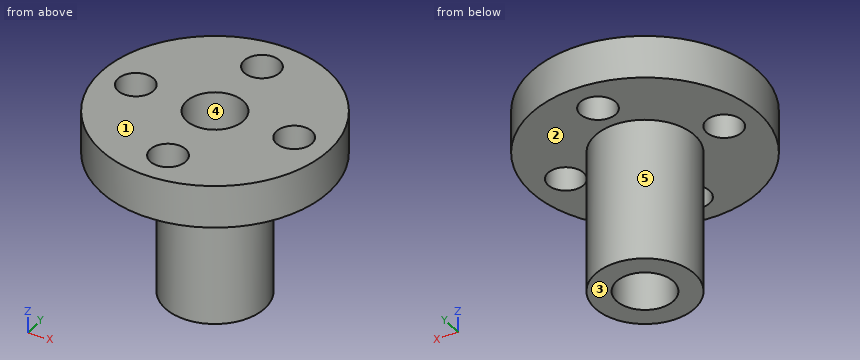
from build123d import *

# Parameters (mm, degrees)
SKETCH1_R           = 8
SKETCH1_R_2         = 1.25
BOSS_EXTRUDE1_DEPTH = 3
SKETCH2_R           = 3.5
BOSS_EXTRUDE2_DEPTH = 10
SKETCH3_R           = 2
CUT_EXTRUDE1_DEPTH  = 18.23368794


with BuildPart() as part:
    # Sketch1 → Boss-Extrude1 (new body)
    with BuildSketch(Plane.XY):
        Circle(SKETCH1_R)
        with Locations((0, 5.5)):
            Circle(SKETCH1_R_2, mode=Mode.SUBTRACT)
        with Locations((5.5, 0)):
            Circle(SKETCH1_R_2, mode=Mode.SUBTRACT)
        with Locations((0, -5.5)):
            Circle(SKETCH1_R_2, mode=Mode.SUBTRACT)
        with Locations((-5.5, 0)):
            Circle(SKETCH1_R_2, mode=Mode.SUBTRACT)
    extrude(amount=BOSS_EXTRUDE1_DEPTH)

    # Sketch2 → Boss-Extrude2 (add)
    with BuildSketch(Plane.XY):
        Circle(SKETCH2_R)
    extrude(amount=-BOSS_EXTRUDE2_DEPTH)

    # Sketch3 → Cut-Extrude1 (cut, through all)
    with BuildSketch(Plane.XY.offset(3)):
        Circle(SKETCH3_R)
    extrude(amount=-CUT_EXTRUDE1_DEPTH, mode=Mode.SUBTRACT)


solid = part.part
For this review, take the finished solid that the model builds, in its own axes (mm). Face numbers are marked on the shaded views. A direction names the side the tool comes from. Give positions to 0.01 mm unless a question says otherwise; leave off trailing zeros. Order: outer loops, then holes, each group sorted by start corner. A loop starts at its lowest first (then second) coordinate and runs counter-clockwise, first axis right, second up. Notation, with made-up numbers: (27, 57.25) - (83, 57.25) arc R24 ccw to (83, 88.25) - close; hole circle Ø9 at (20.25, 16). An arc over 180 degrees is marked (long way). Answer as a JSON object with one key per item and string values. Group by question number.
Item 1: Take a section at C-C on y = -5.5. Give the boundary of the cut face in (x, z), and give its area (3 significant figures).
Item 2: Take a section at A-A on y = 0. Give the boundary of the cut face in (x, z), and give its area (3 significant figures).
Item 3: Wall thickness on line 1 along Y through (x, z) = (0, 1.65); line 2 along Y through (x, z) = (0, -3.5); line 3 along Z through (x, y) = (-3.75, 6.25): over which ranges is each line inside the solid? List them lowest first.
Item 4: Machinability: for the marked faces 1 and 2, which of the approach directions +Z, -Z, +X, -X, +Y, -Y give a long, thin tool a straight path to every point of the face, cutting with its end or side? Answer none if there is none.
Item 5: Draft analysis for pull direction Y (two halves, no side actions). For the marked faces 3, 4 and 5, state which applies: pulls with the +Y half, pulls with the -Y half, needs draft (parallel to the pull), parting line crosses it, or undercut.
Item 6: Clearance check with flat-ended pins moving along their axes: pin 1 Ø8 at (x, y) = (-5, -1.5) entering from -Z; pin 2 Ø3 at (x, z) = (4, -3.5) entering from -Y; pin 3 Ø3 at (x, z) = (-2.5, -5.5) entering from +Y. State where each tip first meets the part, or that it passes through.
Reported:
{
 "1": {"outline": "(-5.81, 0) - (-1.25, 0) - (-1.25, 3) - (-5.81, 3) - close; (1.25, 0) - (5.81, 0) - (5.81, 3) - (1.25, 3) - close", "area": "27.4 mm^2"},
 "2": {"outline": "(-8, 0) - (-6.75, 0) - (-6.75, 3) - (-8, 3) - close; (-4.25, 0) - (-3.5, 0) - (-3.5, -10) - (-2, -10) - (-2, 3) - (-4.25, 3) - close; (2, -10) - (3.5, -10) - (3.5, 0) - (4.25, 0) - (4.25, 3) - (2, 3) - close; (6.75, 0) - (8, 0) - (8, 3) - (6.75, 3) - close", "area": "51.0 mm^2"},
 "3": {"line 1": "-8 to -6.75, -4.25 to -2, 2 to 4.25, 6.75 to 8", "line 2": "-3.5 to -2, 2 to 3.5", "line 3": "0 to 3"},
 "4": {"face 1": "+Z, +X, -X, +Y, -Y", "face 2": "-Z"},
 "5": {"face 3": "needs draft", "face 4": "undercut", "face 5": "parting line crosses it"},
 "6": {"pin 1": "z = -10", "pin 2": "y = -2.45", "pin 3": "y = 3.35"}
}
